Geometry check sheet. Reference: the model listing, model coordinates, mm. Face numbers are marked on the shaded views. A direction names the side the tool comes from. Give positions to 0.01 mm unless a question says otherwise; leave off trailing zeros. Loops run counter-clockwise (first coordinate to the right, second up) from the corner with the lowest first, then second, coordinate; pieces in that order, holes last. Notation, with made-up numbers: (54.5, 53.5) -> (61.5, 53.5) arc R28 ccw to (61.5, 82.5) -> close; hole circle Ø6 at (24.5, 86). An arc over 180 degrees is marked (long way). One line per item, written item: value. Start each with the question number.
(1) Sectioned sample at A-A, the plane x = 1.25. Record the cut outline in (y, z), then the cut area to 3 significant figures.
(2) Tool access check on the marked faces 3, 4 and 5. Record the directions out of +Z, -Z, +X, -X, +Y, -Y that give a thin tool (end or side, any length) a straight path to the whole face; none if there is none.
(3) Draft check along Z on the marked faces 1 and 2. Enter one of: pulls with the +Z half, pulls with the -Z half, needs draft (parallel to the pull), parting line crosses it, or undercut.
(4) Scan lines: line 1 along Z through (x, y) = (-2.3, 0) (3 decimals); line 2 along Z through (x, y) = (-6.5, 0); line 3 along X through (y, z) = (-5.5, -1.75). Record each from-to range of solid material in increasing order. Write a range as from..to.
(5) Gauge pin test, flat ends, axial feed: pin 1 Ø4 at (x, z) = (1.5, 5.5) entering from -Y; pin 2 Ø1.5 at (x, z) = (2.5, 1.5) entering from -Y; pin 3 Ø4 at (x, z) = (-1.5, -2) entering from -Y. Record the tip position at first contact, or that the pin passes through.
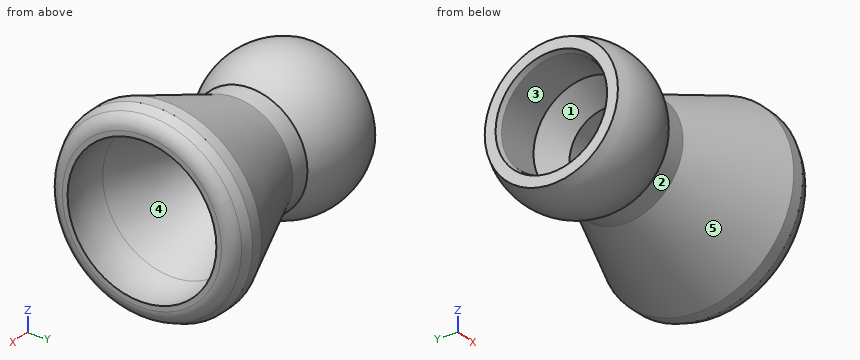
from build123d import *

# Parameters (mm, degrees)
FILLET1_R      = 1.27
CHAMFER1_SIZE  = 0.43942
CHAMFER1_SIZE2 = 0.177537204


with BuildPart() as part:
    # Sketch2 → Revolve1 (revolve)
    with BuildSketch(Plane.XY):
        with BuildLine():
            Line((-9.6139, 5.59308), (-9.6139, 4.5085))
            Line((-9.6139, 4.5085), (-5.482784752, 4.5085))
            Line((-5.482784752, 4.5085), (-3.173095, 3.175))
            Line((-3.173095, 3.175), (-0.77410359, 3.175))
            Line((-0.77410359, 3.175), (6.016717794, 5.918669934))
            ThreePointArc((6.016717794, 5.918669934), (7.790814141, 6.349535218), (9.6139, 6.252474944))
            Line((9.6139, 6.252474944), (9.6139, 7.492691343))
            Line((9.6139, 7.492691343), (8.1153, 8.1915))
            Line((8.1153, 8.1915), (7.099270393, 8.1915))
            Line((7.099270393, 8.1915), (-1.1049, 4.8768))
            Line((-1.1049, 4.8768), (-2.77622, 4.8768))
            ThreePointArc((-2.77622, 4.8768), (-6.088468301, 6.252474944), (-9.6139, 5.59308))
        make_face()
    revolve(axis=Axis((-152.4, 0, 0), (1, 0, 0)))

    # Fillet1
    fillet1_edges = [part.edges().sort_by_distance(p)[0] for p in [
        (9.6139, -7.492691343, 0),
    ]]
    fillet(fillet1_edges, radius=FILLET1_R)

    # Chamfer1
    chamfer1_edges = [part.edges().sort_by_distance(p)[0] for p in [
        (-9.6139, -4.5085, 0),
    ]]
    chamfer1_side = [part.faces().sort_by_distance(p)[0] for p in [
        (-7.548342376, -4.5085, 0),
    ]]
    chamfer(chamfer1_edges, length=CHAMFER1_SIZE, length2=CHAMFER1_SIZE2, reference=chamfer1_side[0])


solid = part.part
Calculated:
1. outline: circle Ø11.66 at (0, 0); hole circle Ø7.99 at (0, 0)
1. area: 56.6 mm2
2. face 3: -X
2. face 4: +X
2. face 5: none
3. face 1: undercut
3. face 2: parting line crosses it
4. line 1: z = -4.877..-3.175, 3.175..4.877
4. line 2: z = -6.28..-4.51, 4.51..6.28
4. line 3: x = -9.24..-4.25, 1.11..5.65
5. pin 1: stops at y = -5.09
5. pin 2: stops at y = -6.5
5. pin 3: stops at y = -5.33
